from build123d import *

# Parameters (mm, degrees)
BOSS_EXTRUDE1_DEPTH = 3.175
CUT_EXTRUDE1_REACH  = 809.569
SKETCH2_W           = 286
SKETCH2_H           = 215


with BuildPart() as part:
    # Sketch1 → Boss-Extrude1 (new body)
    with BuildSketch(Plane(origin=(0, 0, 0), x_dir=(1, 0, 0), z_dir=(0, 1, 0))):
        Polygon((-762, 46.42), (-742.95, 46.42), (-742.95, 8.32), (-762, 8.32), (-762, -267.42), (762, -267.42), (762, 8.32), (742.95, 8.32), (742.95, 46.42), (762, 46.42), (762, 267.42), (-762, 267.42), align=None)
    extrude(amount=BOSS_EXTRUDE1_DEPTH)

    # Sketch2 → Cut-Extrude1 (cut, up to next)
    with BuildSketch(Plane(origin=(0, 3.175, 0), x_dir=(1, 0, 0), z_dir=(0, 1, 0)), mode=Mode.PRIVATE) as cut_extrude1_sk1:
        with Locations((-552, -82.92)):
            Rectangle(SKETCH2_W, SKETCH2_H)
    cut_extrude1_tool1 = extrude(cut_extrude1_sk1.sketch, amount=-CUT_EXTRUDE1_REACH, mode=Mode.PRIVATE) & part.part
    add(cut_extrude1_tool1.solids().sort_by_distance((-552, 3.175, 82.92))[0], mode=Mode.SUBTRACT)


solid = part.part
Could you check a few things on this model? Use its own coordinates, in mm. Give positions to 0.01 mm unless a question says otherwise; leave off trailing zeros. Loops run counter-clockwise (first coordinate to the right, second up) from the corner with the lowest first, then second, coordinate; pieces in that order, holes last. Notation, with made-up numbers: (-7.75, -1.75) -> (11.25, -1.75) arc R32 cw to (11.25, 32.25) -> close; hole circle Ø5 at (50, -33). An arc over 180 degrees is marked (long way). Return JSON: item names as keys, results as strings.
Item 1: I'm going to push a flat-ended pin straight in: pin 1 (1.5 mm diameter, centred on y = 2, z = -18.5, fed in from -X). Where does the tip first touch, or does it pass through?
Geometry results:
{"pin 1": "stops at x = -742.95"}
Item 2: I need wall thicknesses on L1, parallel to X at y = 2.15, z = -21; L2, parallel to X at y = 0.25, z = 121.5; L3, parallel to Z at x = -461.5, y = 1.35. Which ranges of each line are inside material? Lowest first, please. Write a range as from..to.
Geometry results:
{"L1": "x = -742.95..-695, -409..742.95", "L2": "x = -762..-695, -409..762", "L3": "z = -267.42..-24.58, 190.42..267.42"}
Item 3: If we section it at A-A on z = 113.5: List the corners of the cut face in (x, y) for me (3 decimals), plus the area to 3 significant figures.
Geometry results:
{"outline": "(-762, 0) -> (-695, 0) -> (-695, 3.175) -> (-762, 3.175) -> close; (-409, 0) -> (762, 0) -> (762, 3.175) -> (-409, 3.175) -> close", "area": "3,930 mm²"}
Item 4: If we section it at B-B on y = 1.75: List the corners of the cut face in (x, z) for me, plus the area to 3 significant figures.
Geometry results:
{"outline": "(-762, -267.42) -> (762, -267.42) -> (762, -46.42) -> (742.95, -46.42) -> (742.95, -8.32) -> (762, -8.32) -> (762, 267.42) -> (-762, 267.42) -> (-762, -8.32) -> (-742.95, -8.32) -> (-742.95, -46.42) -> (-762, -46.42) -> close; hole (-695, -24.58) -> (-409, -24.58) -> (-409, 190.42) -> (-695, 190.42) -> close", "area": "752,000 mm²"}
